Answer from the drawing. Dimensions are ordinates in mm from the lowest x, y and z of the part. A direction names the side the tool comes from. Give positions to 0.01 mm unless a question says otherwise; leave off trailing zeros. Loops run counter-clockwise (first coordinate to the right, second up) from the corner with the lowest first, then second, coordinate; pieces in that order, holes last.
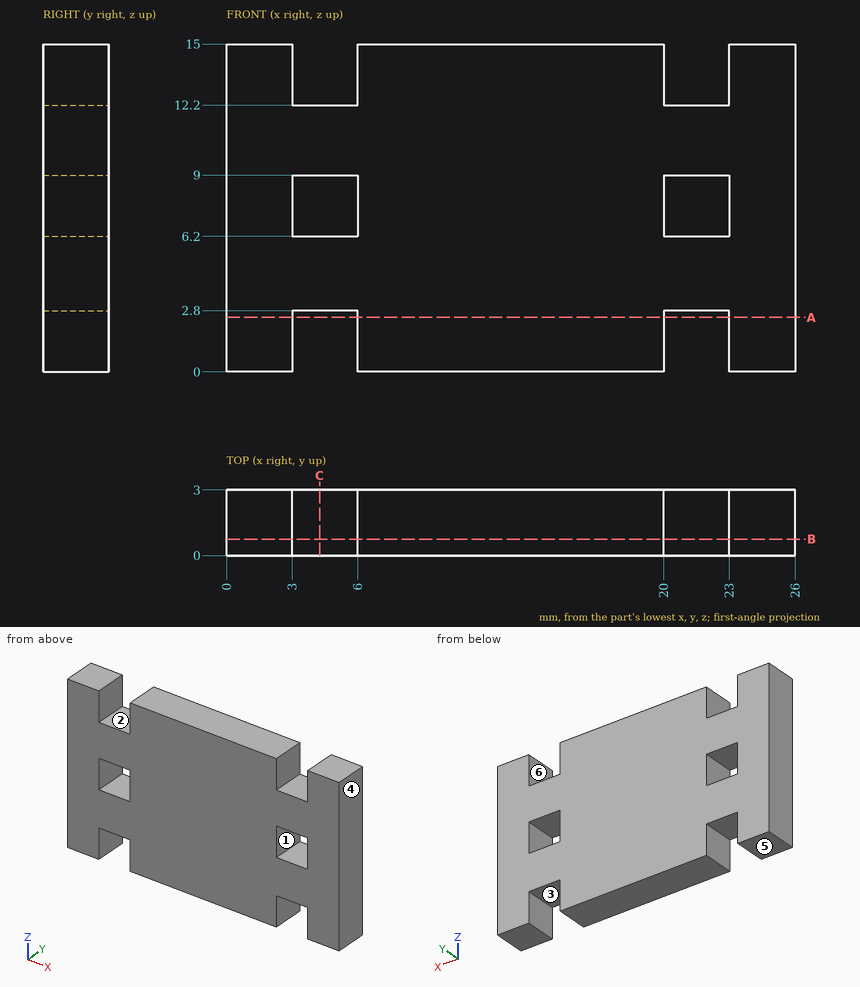
Item 1: Determine the mould class of the marked faces 4, 5 and 6 for opening direction X: released by +X, released by -X, zero draft, split by the parting line, or undercut.
Item 2: Consider line 1 (X direction, y = 1.3, z = 6.25); line 2 (Z direction, x = 4.5, y = 1.1). Determine where each line is inside the solid, lowest interval first.
Item 3: Find section B-B, the plane y = 0.75. Write down the section's boundary in (x, z).
Item 4: Find section A-A, the plane z = 2.5. Write down the section's boundary in (x, y).
Item 5: For the marked faces 1, 2 and 3, determine the directions among +Z, -Z, +X, -X, +Y, -Y from which every point of the face is accessible in a straight line to the end or side of a thin tool.
Item 6: Flat-ended cylindrical pins translate along their axes: pin 1 Ø0.9 at (x, y) = (22, 2) entering from +Z; pin 2 Ø1.4 at (y, z) = (2, 13) entering from -X. Find the tip coordinate at first contact, or state that the pin passes through.
Item 7: Find section C-C, the plane x = 4.25. Write down the section's boundary in (y, z).
Ans:
1. face 4: released by +X
1. face 5: zero draft
1. face 6: undercut
2. line 1: x = 0 to 3, 6 to 20, 23 to 26
2. line 2: z = 2.8 to 6.2, 9 to 12.2
3. outline: (0, 0) - (3, 0) - (3, 2.8) - (6, 2.8) - (6, 0) - (20, 0) - (20, 2.8) - (23, 2.8) - (23, 0) - (26, 0) - (26, 15) - (23, 15) - (23, 12.2) - (20, 12.2) - (20, 15) - (6, 15) - (6, 12.2) - (3, 12.2) - (3, 15) - (0, 15) - close; hole (3, 6.2) - (6, 6.2) - (6, 9) - (3, 9) - close; hole (20, 6.2) - (23, 6.2) - (23, 9) - (20, 9) - close
4. outline: (0, 0) - (3, 0) - (3, 3) - (0, 3) - close; (6, 0) - (20, 0) - (20, 3) - (6, 3) - close; (23, 0) - (26, 0) - (26, 3) - (23, 3) - close
5. face 1: +Y, -Y
5. face 2: +Z, +Y, -Y
5. face 3: -Z, +Y, -Y
6. pin 1: stops at z = 12.2
6. pin 2: stops at x = 0
7. outline: (0, 2.8) - (3, 2.8) - (3, 6.2) - (0, 6.2) - close; (0, 9) - (3, 9) - (3, 12.2) - (0, 12.2) - close
